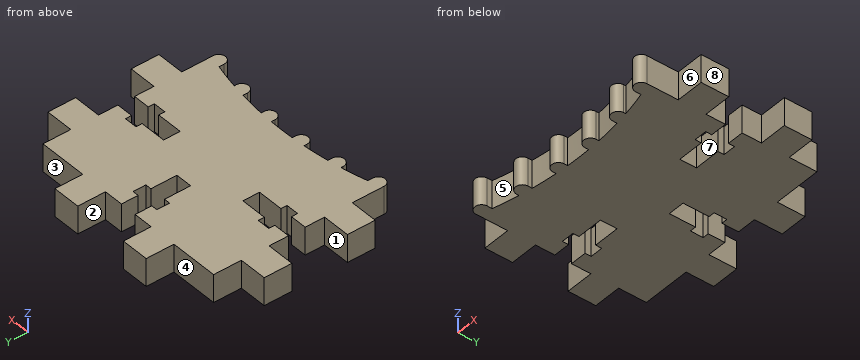
from build123d import *

# Parameters (mm, degrees)
BOSS_EXTRUDE1_DEPTH = 5


with BuildPart() as part:
    # Sketch1 → Boss-Extrude1 (new body)
    with BuildSketch(Plane.XY):
        with BuildLine():
            Line((-18.7, 12.184100059), (-18.7, 11.940969848))
            ThreePointArc((-18.7, 11.940969848), (-17.5, 10.740969848), (-16.3, 11.940969848))
            Line((-16.3, 11.940969848), (-16.3, 12.872306458))
            ThreePointArc((-16.3, 12.872306458), (-14.009663332, 13.435283428), (-11.7, 13.912819196))
            Line((-11.7, 13.912819196), (-11.7, 13.525873247))
            ThreePointArc((-11.7, 13.525873247), (-10.5, 12.325873247), (-9.3, 13.525873247))
            Line((-9.3, 13.525873247), (-9.3, 14.315284764))
            ThreePointArc((-9.3, 14.315284764), (-7.004652926, 14.612477668), (-4.7, 14.825824116))
            Line((-4.7, 14.825824116), (-4.7, 14.303469937))
            ThreePointArc((-4.7, 14.303469937), (-3.5, 13.103469937), (-2.3, 14.303469937))
            Line((-2.3, 14.303469937), (-2.3, 14.958332786))
            ThreePointArc((-2.3, 14.958332786), (0, 15), (2.3, 14.958332786))
            Line((2.3, 14.958332786), (2.3, 14.303469937))
            ThreePointArc((2.3, 14.303469937), (3.5, 13.103469937), (4.7, 14.303469937))
            Line((4.7, 14.303469937), (4.7, 14.825824116))
            ThreePointArc((4.7, 14.825824116), (7.004652926, 14.612477668), (9.3, 14.315284764))
            Line((9.3, 14.315284764), (9.3, 13.525873247))
            ThreePointArc((9.3, 13.525873247), (10.5, 12.325873247), (11.7, 13.525873247))
            Line((11.7, 13.525873247), (11.7, 13.912819196))
            ThreePointArc((11.7, 13.912819196), (14.009663332, 13.435283428), (16.3, 12.872306458))
            Line((16.3, 12.872306458), (16.3, 11.940969848))
            ThreePointArc((16.3, 11.940969848), (17.5, 10.740969848), (18.7, 11.940969848))
            Line((18.7, 11.940969848), (18.7, 12.184100059))
            Line((18.7, 12.184100059), (18.7, 17.622423299))
            Line((18.7, 17.622423299), (23.7, 17.622423299))
            Line((23.7, 17.622423299), (23.7, 22.622423299))
            Line((23.7, 22.622423299), (18.7, 22.622423299))
            Line((18.7, 22.622423299), (18.7, 26.122423299))
            Line((18.7, 26.122423299), (15.7, 26.122423299))
            Line((15.7, 26.122423299), (15.7, 25.022423299))
            Line((15.7, 25.022423299), (13.4, 25.022423299))
            Line((13.4, 25.022423299), (13.4, 26.122423299))
            Line((13.4, 26.122423299), (8.7, 26.122423299))
            Line((8.7, 26.122423299), (8.7, 29.122423299))
            Line((8.7, 29.122423299), (13.4, 29.122423299))
            Line((13.4, 29.122423299), (13.4, 30.222423299))
            Line((13.4, 30.222423299), (15.7, 30.222423299))
            Line((15.7, 30.222423299), (15.7, 29.122423299))
            Line((15.7, 29.122423299), (18.7, 29.122423299))
            Line((18.7, 29.122423299), (18.7, 32.622423299))
            Line((18.7, 32.622423299), (23.7, 32.622423299))
            Line((23.7, 32.622423299), (23.7, 37.622423299))
            Line((23.7, 37.622423299), (18.7, 37.622423299))
            Line((18.7, 37.622423299), (18.7, 42.622423299))
            Line((18.7, 42.622423299), (10, 42.622423299))
            Line((10, 42.622423299), (10, 47.622423299))
            Line((10, 47.622423299), (5, 47.622423299))
            Line((5, 47.622423299), (5, 42.622423299))
            Line((5, 42.622423299), (1.5, 42.622423299))
            Line((1.5, 42.622423299), (1.5, 39.622423299))
            Line((1.5, 39.622423299), (2.6, 39.622423299))
            Line((2.6, 39.622423299), (2.6, 37.322423299))
            Line((2.6, 37.322423299), (1.5, 37.322423299))
            Line((1.5, 37.322423299), (1.5, 32.622423299))
            Line((1.5, 32.622423299), (-1.5, 32.622423299))
            Line((-1.5, 32.622423299), (-1.5, 37.322423299))
            Line((-1.5, 37.322423299), (-2.6, 37.322423299))
            Line((-2.6, 37.322423299), (-2.6, 39.622423299))
            Line((-2.6, 39.622423299), (-1.5, 39.622423299))
            Line((-1.5, 39.622423299), (-1.5, 42.622423299))
            Line((-1.5, 42.622423299), (-5, 42.622423299))
            Line((-5, 42.622423299), (-5, 47.622423299))
            Line((-5, 47.622423299), (-10, 47.622423299))
            Line((-10, 47.622423299), (-10, 42.622423299))
            Line((-10, 42.622423299), (-18.7, 42.622423299))
            Line((-18.7, 42.622423299), (-18.7, 37.622423299))
            Line((-18.7, 37.622423299), (-23.7, 37.622423299))
            Line((-23.7, 37.622423299), (-23.7, 32.622423299))
            Line((-23.7, 32.622423299), (-18.7, 32.622423299))
            Line((-18.7, 32.622423299), (-18.7, 29.122423299))
            Line((-18.7, 29.122423299), (-15.7, 29.122423299))
            Line((-15.7, 29.122423299), (-15.7, 30.222423299))
            Line((-15.7, 30.222423299), (-13.4, 30.222423299))
            Line((-13.4, 30.222423299), (-13.4, 29.122423299))
            Line((-13.4, 29.122423299), (-8.7, 29.122423299))
            Line((-8.7, 29.122423299), (-8.7, 26.122423299))
            Line((-8.7, 26.122423299), (-13.4, 26.122423299))
            Line((-13.4, 26.122423299), (-13.4, 25.022423299))
            Line((-13.4, 25.022423299), (-15.7, 25.022423299))
            Line((-15.7, 25.022423299), (-15.7, 26.122423299))
            Line((-15.7, 26.122423299), (-18.7, 26.122423299))
            Line((-18.7, 26.122423299), (-18.7, 22.622423299))
            Line((-18.7, 22.622423299), (-23.7, 22.622423299))
            Line((-23.7, 22.622423299), (-23.7, 17.622423299))
            Line((-23.7, 17.622423299), (-18.7, 17.622423299))
            Line((-18.7, 17.622423299), (-18.7, 12.184100059))
        make_face()
    extrude(amount=BOSS_EXTRUDE1_DEPTH)


solid = part.part
The listing builds one solid part. Answer for the finished solid, in the listing's coordinates (mm). Face numbers are marked on the shaded views. A direction names the side the tool comes from. Round coordinates to 2 decimals unless told otherwise and drop trailing zeros. Write each loop counter-clockwise with the first axis right and the second up, starting at its lowest first coordinate (ties: lowest second). Pieces come first, ordered by that corner, then holes. Notation, with made-up numbers: M 24.25,49.25 L 59.25,49.25 A25 ccw 59.25,68.25 Z; hole C -11,68 d10. An arc over 180 degrees is marked long. Write each question's results on one line, items separated by ' | '. Start each with the question number.
Item 1: A cutting plane is placed at D-D on x = -0.5. Write down the section's boundary in (y, z), and give its area (3 significant figures).
Item 2: For a pull along Y with two mould halves and no side action, classify the marked faces 6, 7 and 8 as pulls with the +Y half, pulls with the -Y half, needs draft (parallel to the pull), parting line crosses it, or undercut.
Item 3: Straight lines are drawn through the part: L1, parallel to X at y = 26, z = 0.55; L2, parallel to X at y = 36.5, z = 4.05; L3, parallel to X at y = 12, z = 2.1. For each, find the intervals that lie inside material, in ascending order. Write a range as [from, to].
Item 4: A cutting plane is placed at A-A on x = 10.5. Write down the section's boundary in (y, z).
Item 5: For the marked faces 1, 2, 3, 4 and 5, determine the directions among +Z, -Z, +X, -X, +Y, -Y from which every point of the face is accessible in a straight line to the end or side of a thin tool.
Item 6: A cutting plane is placed at C-C on y = 31. Write down the section's boundary in (x, z), and give its area (3 significant figures).
Item 7: A cutting plane is placed at B-B on x = -20.5. Write down the section's boundary in (y, z), and give its area (3 significant figures).
Item 8: Flat-ended cylindrical pins translate along their axes: pin 1 Ø0.5 at (y, z) = (30, 3.5) entering from -X; pin 2 Ø1.5 at (x, z) = (-16, 2) entering from +Y; pin 3 Ø1.5 at (x, z) = (-22.5, 1.5) entering from -Y; pin 4 Ø3 at (x, y) = (4, 18.5) entering from -Z. Find the tip coordinate at first contact, or state that the pin passes through.
Check sheet entries:
1) outline: M 15,0 L 32.62,0 L 32.62,5 L 15,5 Z | area: 88.1 mm²
2) face 6: pulls with the -Y half | face 7: undercut | face 8: needs draft
3) L1: [-18.7, -15.7], [-13.4, 13.4], [15.7, 18.7] | L2: [-23.7, -1.5], [1.5, 23.7] | L3: [-18.7, -16.3], [16.3, 18.7]
4) outline: M 12.33,0 L 26.12,0 L 26.12,5 L 12.33,5 Z; M 29.12,0 L 42.62,0 L 42.62,5 L 29.12,5 Z
5) face 1: +Z, -Z, -X | face 2: +Z, -Z, +Y | face 3: +Z, -Z, +X, +Y | face 4: +Z, -Z, -X, +Y | face 5: +Z, -Z, -Y
6) outline: M -18.7,0 L 18.7,0 L 18.7,5 L -18.7,5 Z | area: 187 mm²
7) outline: M 17.62,0 L 22.62,0 L 22.62,5 L 17.62,5 Z; M 32.62,0 L 37.62,0 L 37.62,5 L 32.62,5 Z | area: 50.0 mm²
8) pin 1: x = -18.7 | pin 2: y = 42.62 | pin 3: y = 17.62 | pin 4: z = 0
